Geometry check sheet. Reference: the model listing, model coordinates, mm. Give positions to 0.01 mm unless a question says otherwise; leave off trailing zeros. Write each loop counter-clockwise with the first axis right and the second up, starting at its lowest first coordinate (ties: lowest second). Pieces come first, ordered by that corner, then holes. Notation, with made-up numbers: (60, -19) -> (71, -19) arc R19 ccw to (71, 4) -> close; hole circle Ø8 at (5, 39). An arc over 180 degrees is marked (long way). One line per item, written item: value.
from build123d import *

# Parameters (mm, degrees)
SKETCH_1_W               = 140
SKETCH_1_H               = 80
EXTRUDE_1_DEPTH          = 3
SKETCH_2_R               = 2.1
CUT_EXTRUDE_1_DEPTH      = 81.678373806
CUT_EXTRUDE_2_DEPTH      = 81.678373806
CUT_EXTRUDE_2_DEPTH_BACK = 81.678373806
SKETCH_3_R               = 1.25
CUT_EXTRUDE_3_DEPTH      = 81.678373806
CUT_EXTRUDE_3_DEPTH_BACK = 81.678373806
SKETCH_4_R               = 12.5


with BuildPart() as part:
    # 草图1 → 凸台-拉伸1 (new body)
    with BuildSketch(Plane.XY):
        Rectangle(SKETCH_1_W, SKETCH_1_H)
    extrude(amount=EXTRUDE_1_DEPTH)

    # 草图2 → 切除-拉伸1 (cut, through all)
    with BuildSketch(Plane.XY.offset(3)):
        with Locations((-60, 30)):
            Circle(SKETCH_2_R)
        with Locations((-30, 30)):
            Circle(SKETCH_2_R)
        with Locations((0, 30)):
            Circle(SKETCH_2_R)
        with Locations((30, 30)):
            Circle(SKETCH_2_R)
        with Locations((60, 30)):
            Circle(SKETCH_2_R)
        with Locations((-60, 0)):
            Circle(SKETCH_2_R)
        with Locations((-60, -30)):
            Circle(SKETCH_2_R)
        with Locations((-60, -60)):
            Circle(SKETCH_2_R)
        with Locations((-60, -90)):
            Circle(SKETCH_2_R)
        with Locations((-60, -120)):
            Circle(SKETCH_2_R)
        with Locations((-60, -150)):
            Circle(SKETCH_2_R)
        with Locations((-60, -180)):
            Circle(SKETCH_2_R)
        with Locations((-60, -210)):
            Circle(SKETCH_2_R)
        with Locations((60, -210)):
            Circle(SKETCH_2_R)
        with Locations((60, -180)):
            Circle(SKETCH_2_R)
        with Locations((60, -150)):
            Circle(SKETCH_2_R)
        with Locations((60, -120)):
            Circle(SKETCH_2_R)
        with Locations((60, -90)):
            Circle(SKETCH_2_R)
        with Locations((60, -60)):
            Circle(SKETCH_2_R)
        with Locations(Location((60, -30, 0), (0, 0, 180))):
            Circle(SKETCH_2_R)
        with Locations(Location((60, 0, 0), (0, 0, 180))):
            Circle(SKETCH_2_R)
        with Locations(Location((30, -30, 0), (0, 0, 180))):
            Circle(SKETCH_2_R)
        with Locations(Location((0, -30, 0), (0, 0, 180))):
            Circle(SKETCH_2_R)
        with Locations(Location((-30, -30, 0), (0, 0, 180))):
            Circle(SKETCH_2_R)
    extrude(amount=-CUT_EXTRUDE_1_DEPTH, mode=Mode.SUBTRACT)

    # 草图3 → 切除-拉伸2 (cut, two sides: drawn at the far end of the back side and taken through both)
    with BuildSketch(Plane(origin=(0, 0, 0), x_dir=(-1, 0, 0), z_dir=(0, 0, -1)).offset(-CUT_EXTRUDE_2_DEPTH_BACK)):
        with Locations((19, 0)):
            Circle(SKETCH_3_R)
        with Locations((0, -19)):
            Circle(SKETCH_3_R)
        with Locations((-19, 0)):
            Circle(SKETCH_3_R)
        with Locations((0, 19)):
            Circle(SKETCH_3_R)
    extrude(amount=CUT_EXTRUDE_2_DEPTH + CUT_EXTRUDE_2_DEPTH_BACK, mode=Mode.SUBTRACT)

    # 草图4 → 切除-拉伸3 (cut, two sides: drawn at the far end of the back side and taken through both)
    with BuildSketch(Plane(origin=(0, 0, 0), x_dir=(-1, 0, 0), z_dir=(0, 0, -1)).offset(-CUT_EXTRUDE_3_DEPTH_BACK)):
        Circle(SKETCH_4_R)
    extrude(amount=CUT_EXTRUDE_3_DEPTH + CUT_EXTRUDE_3_DEPTH_BACK, mode=Mode.SUBTRACT)


solid = part.part
1) Depth check by flat-ended pin: pin 1 Ø15 at (x, y) = (0, 0) entering from +Z. Enter the tip coordinate at first touch or a pass-through.
Verdict:
pin 1: through
2) Sectioned sample at A-A on y = -30. Record the cut outline in (x, z), plus the area to 3 significant figures.
Verdict:
outline: (-70, 0) -> (-62.1, 0) -> (-62.1, 3) -> (-70, 3) -> close; (-57.9, 0) -> (-32.1, 0) -> (-32.1, 3) -> (-57.9, 3) -> close; (-27.9, 0) -> (-2.1, 0) -> (-2.1, 3) -> (-27.9, 3) -> close; (2.1, 0) -> (27.9, 0) -> (27.9, 3) -> (2.1, 3) -> close; (32.1, 0) -> (57.9, 0) -> (57.9, 3) -> (32.1, 3) -> close; (62.1, 0) -> (70, 0) -> (70, 3) -> (62.1, 3) -> close
area: 357 mm^2
3) Sectioned sample at C-C on y = -5. Record the cut outline in (x, z).
Verdict:
outline: (-70, 0) -> (-11.46, 0) -> (-11.46, 3) -> (-70, 3) -> close; (11.46, 0) -> (70, 0) -> (70, 3) -> (11.46, 3) -> close
4) Scan lines: probe 1 along Y at (x, z) = (30, 2.3); probe 2 along Y at (x, z) = (-60, 0.75); probe 3 along X at (y, z) = (19, 2.45). Record each from-to range of solid material in increasing order.
Verdict:
probe 1: -40 to -32.1, -27.9 to 27.9, 32.1 to 40
probe 2: -40 to -32.1, -27.9 to -2.1, 2.1 to 27.9, 32.1 to 40
probe 3: -70 to -1.25, 1.25 to 70
5) Sectioned sample at B-B on z = 1.9. Give the number of separate pieces and of enclosed holes in the cut face, plus the area to 3 significant figures.
Verdict:
separate pieces: 1
enclosed holes: 17
area: 10,500 mm^2
